from build123d import *

# Parameters (mm, degrees)
F0_R     = 3.81
F1_DEPTH = 6.35
F2_T     = -33.02
F3_DEPTH = 7.62


with BuildPart() as f1:
    # F0 (on Front) → F1 (new body, symmetric)
    with BuildSketch(Plane.XZ):
        with BuildLine():
            ThreePointArc((-38.1, 1.128e-07), (-5.64e-08, -38.1), (38.1, 0))
            ThreePointArc((38.1, 0), (5.64e-08, 38.1), (-38.1, 1.128e-07))
        make_face()
        with BuildLine():
            ThreePointArc((-30.48, 0), (-34.2900000564, -3.81), (-38.1, 1.128e-07))
            ThreePointArc((-38.1, 1.128e-07), (-34.2899999436, 3.81), (-30.48, 0))
        make_face(mode=Mode.SUBTRACT)
        with Locations((34.29, 0)):
            Circle(F0_R, mode=Mode.SUBTRACT)
        with BuildLine():
            ThreePointArc((-30.48, 0), (-34.2899999436, 3.81), (-38.1, 1.128e-07))
            ThreePointArc((-38.1, 1.128e-07), (-34.2900000564, -3.81), (-30.48, 0))
        make_face()
        with Locations((34.29, 0)):
            Circle(F0_R)
    extrude(amount=F1_DEPTH, both=True)

    # F2
    f2_openings = [f1.faces().sort_by_distance(p)[0] for p in [
        (0, -6.35, 0),
        (0, 6.35, 0),
    ]]
    offset(amount=F2_T, openings=f2_openings)

    # F0 (on Front) → F3 (join)
    with BuildSketch(Plane.XZ):
        with BuildLine():
            ThreePointArc((-30.48, 0), (-34.2899999436, 3.81), (-38.1, 1.128e-07))
            ThreePointArc((-38.1, 1.128e-07), (-34.2900000564, -3.81), (-30.48, 0))
        make_face()
    extrude(amount=F3_DEPTH)


solid = f1.part
The listing builds one solid part. Answer for the finished solid, in the listing's coordinates (mm). A direction names the side the tool comes from. Round coordinates to 2 decimals unless told otherwise and drop trailing zeros. Order: outer loops, then holes, each group sorted by start corner. A loop starts at its lowest first (then second) coordinate and runs counter-clockwise, first axis right, second up. Notation, with made-up numbers: (25.25, 43.25) -> (29.25, 43.25) arc R25 ccw to (29.25, 66.25) -> close; hole circle Ø1 at (54, -8). An arc over 180 degrees is marked (long way). Put each result on its own line as item: value.
Q1. Section B-B, the plane y = 3 is taken. Write down the section's boundary in (x, z), and give its area (3 significant figures).
Results list:
outline: circle Ø76.2 at (0, 0); hole circle Ø10.16 at (0, 0)
area: 4,480 mm^2
Q2. Section C-C, the plane x = -32 is taken. Write down the section's boundary in (y, z) (3 decimals), and give its area (3 significant figures).
Results list:
outline: (-7.62, -3.045) -> (-6.35, -3.045) -> (-6.35, -20.679) -> (6.35, -20.679) -> (6.35, 20.679) -> (-6.35, 20.679) -> (-6.35, 3.045) -> (-7.62, 3.045) -> close
area: 533 mm^2
Q3. Consider line 1 along Z through (x, y) = (0, 2.5); line 2 along Y through (x, z) = (-7.5, -9.5); line 3 along Z through (x, y) = (-3, 5.5). Determine where each line is inside the solid, lowest interval first.
Results list:
line 1: -38.1 to -5.08, 5.08 to 38.1
line 2: -6.35 to 6.35
line 3: -37.98 to -4.1, 4.1 to 37.98
Q4. Determine the mould class of faces 3 (the cylindrical face through (-30.235, -0.089, -23.183)), 4 (the flat face through (8, -6.35, 1)), 5 (the cylindrical face through (-0.661, -0.089, 5.037)) for opening direction Z: pulls with the +Z half, pulls with the -Z half, needs draft (parallel to the pull), parting line crosses it, or undercut.
Results list:
face 3: parting line crosses it
face 4: needs draft
face 5: undercut
Q5. Section A-A, the plane x = 0 is taken. Write down the section's boundary in (y, z), and give its area (3 significant figures).
Results list:
outline: (-6.35, -38.1) -> (6.35, -38.1) -> (6.35, -5.08) -> (-6.35, -5.08) -> close; (-6.35, 5.08) -> (6.35, 5.08) -> (6.35, 38.1) -> (-6.35, 38.1) -> close
area: 839 mm^2
Q6. Which of the six approach directions +Z, -Z, +X, -X, +Y, -Y give full straight-line access (tool end or side, diameter ignored) to faces 1 (the cylindrical face through (-31.27, -6.98, 2.32)), 2 (the flat face through (8, 6.35, 1))?
Results list:
face 1: -Y
face 2: +Z, -Z, +X, -X, +Y
Q7. Section D-D, the plane z = 18 is taken. Write down the section's boundary in (x, y), and give its area (3 significant figures).
Results list:
outline: (-33.58, -6.35) -> (33.58, -6.35) -> (33.58, 6.35) -> (-33.58, 6.35) -> close
area: 853 mm^2
Q8. Each of these flat-tipped pins is pushed along its axis until it touches: P1, Ø4, axis at x = 20.5, z = 24.5, coming from the -Y side; P2, Ø5, axis at x = -29.5, y = -0.5, coming from the +Z side; P3, Ø16.5, axis at x = 0, z = 0, coming from the +Y side; P4, Ø8, axis at y = -5.5, z = -13, coming from the +X side. Where does it stop, or does it pass through?
Results list:
P1: y = -6.35
P2: z = 26.88
P3: y = 6.35
P4: x = 37.02
